Print and shaded views of the part. All mm, measured from the part's lowest x, y and z. Give positions to 0.01 mm unless a question says otherwise; leave off trailing zeros. Loops run counter-clockwise (first coordinate to the right, second up) from the corner with the lowest first, then second, coordinate; pieces in that order, holes last. Notation, with made-up numbers: (-21.75, -6.75) -> (-2.75, -6.75) arc R20 cw to (-2.75, 6.25) -> close; hole circle Ø5 at (27.25, -22.75). An arc over 180 degrees is marked (long way). Answer as a JSON object with one key per item and string values. Group by question number.
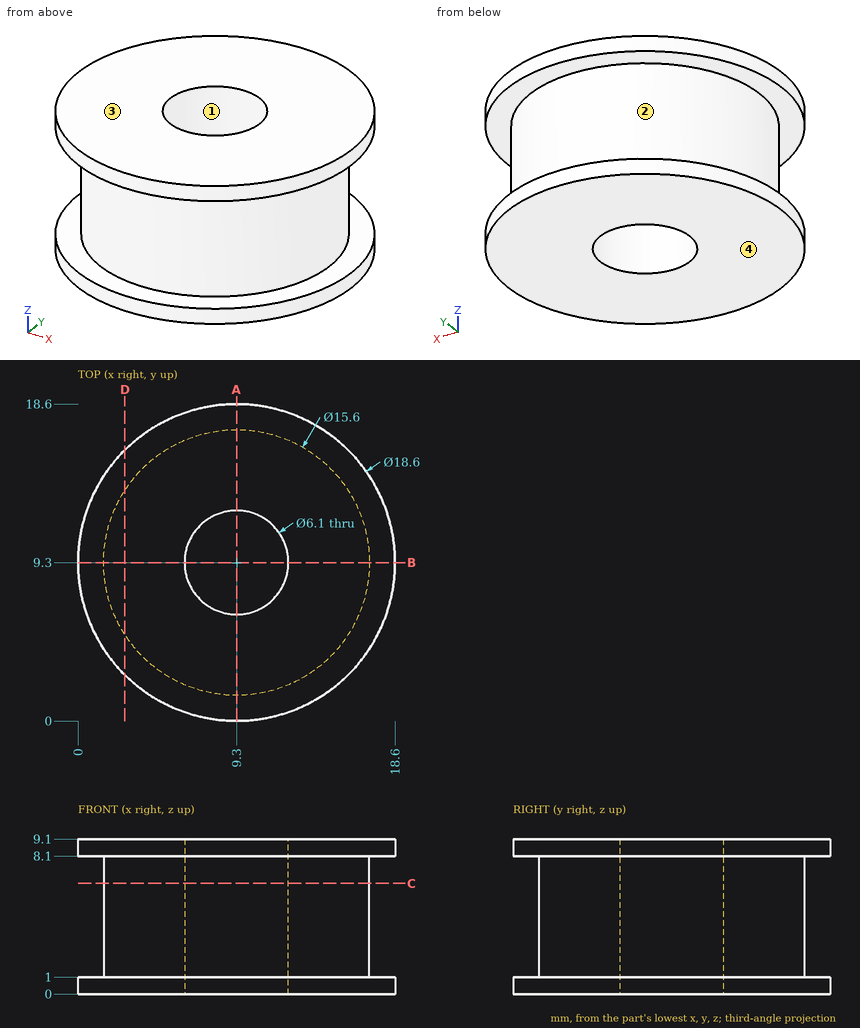
(1) Saw through at A-A on x = 9.3. List the corners of the cut face in (y, z), plus the area to 4 significant figures.
(2) Pin check, flat tips, straight feed: pin 1 (1 mm diameter, centred on y = 8.5, z = 6, fed in from +X); pin 2 (5 mm diameter, centred on x = 11.5, z = 6, fed in from +Y); pin 3 (4 mm diameter, centred on y = 7, z = 7.5, fed in from +X). Stop position of each tip, or through.
(3) Pull direction Z, two halves, no side cores. Call the marked faces 1, 2, 3 and 4: pulls with the +Z half, pulls with the -Z half, needs draft (parallel to the pull), parting line crosses it, or undercut.
(4) Saw through at D-D on x = 2.75. List the corners of the cut face in (y, z), plus the area to 3 significant figures.
(5) Probe line 1 along Y through (x, z) = (9.3, 6.25); line 2 along Y through (x, z) = (8.5, 2.5); line 3 along Y through (x, z) = (15.75, 7.5). List the from-to ranges inside material, lowest first. Write a range as [from, to].
(6) Saw through at C-C on z = 6.5. List the corners of the cut face in (x, y), plus the area to 3 significant figures.
Calculated:
{
 "1": {"outline": "(0, 0) -> (6.25, 0) -> (6.25, 9.1) -> (0, 9.1) -> (0, 8.1) -> (1.5, 8.1) -> (1.5, 1) -> (0, 1) -> close; (12.35, 0) -> (18.6, 0) -> (18.6, 1) -> (17.1, 1) -> (17.1, 8.1) -> (18.6, 8.1) -> (18.6, 9.1) -> (12.35, 9.1) -> close", "area": "92.45 mm^2"},
 "2": {"pin 1": "stops at x = 17.09", "pin 2": "stops at y = 18.56", "pin 3": "stops at x = 18.59"},
 "3": {"face 1": "needs draft", "face 2": "undercut", "face 3": "pulls with the +Z half", "face 4": "pulls with the -Z half"},
 "4": {"outline": "(2.7, 0) -> (15.9, 0) -> (15.9, 1) -> (13.54, 1) -> (13.54, 8.1) -> (15.9, 8.1) -> (15.9, 9.1) -> (2.7, 9.1) -> (2.7, 8.1) -> (5.06, 8.1) -> (5.06, 1) -> (2.7, 1) -> close", "area": "86.5 mm^2"},
 "5": {"line 1": "y = [1.5, 6.25], [12.35, 17.1]", "line 2": "y = [1.54, 6.36], [12.24, 17.06]", "line 3": "y = [4.91, 13.69]"},
 "6": {"outline": "circle Ø15.6 at (9.3, 9.3); hole circle Ø6.1 at (9.3, 9.3)", "area": "162 mm^2"}
}
